from build123d import *

# Parameters (mm, degrees)
F0_W     = 250
F0_H     = 130
F2_DEPTH = 2
F3_DEPTH = 130
F4_R     = 59.99999
F6_DEPTH = 47


# Not quite as in the source:
# - a fillet or chamfer is up to 0.001 mm smaller than in the source, because OpenCascade refuses the exact size


with BuildPart() as f2:
    # F0 (on Top) → F2 (new body)
    with BuildSketch(Plane.XY):
        with Locations((-125, -65)):
            Rectangle(F0_W, F0_H)
    extrude(amount=-F2_DEPTH)

    # F1 (on Front) → F3 (join)
    with BuildSketch(Plane.XZ):
        with BuildLine():
            Line((-67.4997093476, 0), (-65.2703463938, 0))
            ThreePointArc((-65.2703463938, 0), (-125.2703463938, 60), (-185.2703463938, 0))
            Line((-185.2703463938, 0), (-183.04098344, 0))
            ThreePointArc((-183.04098344, 0), (-125.2703463938, 57.7706370462), (-67.4997093476, 0))
        make_face()
        with BuildLine():
            Line((-183.04098344, 0), (-67.4997093476, 0))
            ThreePointArc((-67.4997093476, 0), (-125.2703463938, 57.7706370462), (-183.04098344, 0))
        make_face()
    extrude(amount=F3_DEPTH)

    # F4 (radius 60 in the source; OpenCascade refuses exactly that, so slightly less here)
    f4_edges = [f2.edges().sort_by_distance(p)[0] for p in [
        (-125.270346, -130, 60),
    ]]
    fillet(f4_edges, radius=F4_R)

    # F5 (on Front) → F6 (cut)
    with BuildSketch(Plane.XZ):
        with BuildLine():
            Line((-183.5164714, 0), (-66.640497432, 0))
            ThreePointArc((-66.640497432, 0), (-125.078484416, 58.437986984), (-183.5164714, 0))
        make_face()
    extrude(amount=F6_DEPTH, mode=Mode.SUBTRACT)


solid = f2.part
Input: part model. Units: mm. Frame: model coordinates. A direction names the side the tool comes from. Coordinates: 2 decimals unless noted, no trailing zeros. Loops run counter-clockwise (first coordinate to the right, second up) from the corner with the lowest first, then second, coordinate; pieces in that order, holes last.
Q1. Draft query along X for faces 3 (the face through (-36, -64, 0)), 4 (the face through (-123.793, -23.171, 58.424)), 5 (the face through (-123.951, -34.51, 59.985)). Return one class per face: +X half, -X half, draft (parallel to the pull), parting line (faces both ways), or undercut.
Q2. Material intervals for line 1 (Z direction, x = -23, y = -7.5); line 2 (X direction, y = -10.5, z = 11); line 3 (X direction, y = -31.5, z = 15.5), sorted ascending.
Q3. Cut plane B-B (x = -196.5). Output: boundary loops of the cut face in (y, z).
Q4. Cut plane A-A (y = -20). Output: boundary loops of the cut face in (x, z).
Q5. Set-up query: faces 1 (the face through (-126, -47, 23)), 2 (the face through (-126, 0, -1)). Return all of +Z, -Z, +X, -X, +Y, -Y with unobstructed straight access to the full face (end or side cutting, diameter ignored); none if empty.
Q6. Contact query for flat-ended pins moving along their axis: pin 1 (8 mm diameter, centred on y = -70.5, z = 45, fed in from +X); pin 2 (1.5 mm diameter, centred on y = -28.5, z = 31.5, fed in from -X); pin 3 (2 mm diameter, centred on x = -151, z = 20, fed in from +Y). Output: stop coordinate, or through.
Working result:
1. face 3: draft
1. face 4: undercut
1. face 5: parting line
2. line 1: z = -2 to 0
2. line 2: x = -184.25 to -182.47, -67.69 to -66.29
2. line 3: x = -183.23 to -181.42, -68.73 to -67.31
3. outline: (-130, -2) - (0, -2) - (0, 0) - (-130, 0) - close
4. outline: (-250, -2) - (0, -2) - (0, 0) - (-65.27, 0) arc R60 ccw to (-185.27, 0) - (-250, 0) - close; hole (-183.52, 0) - (-66.64, 0) arc R58.44 ccw to start
5. face 1: +Y
5. face 2: +Z, -Z, +X, -X, +Y
6. pin 1: stops at x = -81.47
6. pin 2: stops at x = -176.79
6. pin 3: stops at y = -47
